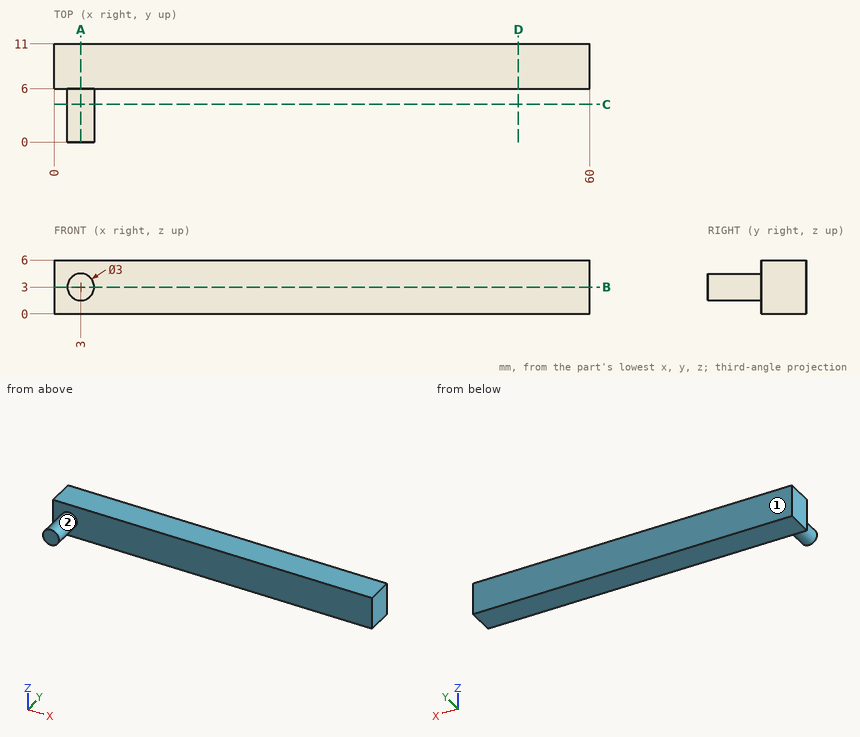
Input: dimensioned drawing with shaded views. Units: mm. Origin: part minimum x, y, z. A direction names the side the tool comes from. Give positions to 0.01 mm unless a question says otherwise; leave off trailing zeros. Order: outer loops, then holes, each group sorted by start corner. A loop starts at its lowest first (then second) coordinate and runs counter-clockwise, first axis right, second up. Notation, with made-up numbers: (-39, -15) -> (9, -15) arc R6 cw to (9, -9) -> close; hole circle Ø9 at (46, 19). An arc over 180 degrees is marked (long way). Use one line per item in the form item = value.
1) Section B-B, the plane z = 3. Return loops of the section in (x, y).
Response values:
outline = (0, 6) -> (1.5, 6) -> (1.5, 0) -> (4.5, 0) -> (4.5, 6) -> (60, 6) -> (60, 11) -> (0, 11) -> close
2) Line query: probe 1 along Y at (x, z) = (27, 1.6); probe 2 along Z at (x, y) = (4, 1.5); probe 3 along X at (y, z) = (2, 3.3). Output: solid intervals per line, ascending.
Response values:
probe_1 = 6 to 11
probe_2 = 1.88 to 4.12
probe_3 = 1.53 to 4.47
3) Section C-C, the plane y = 4.25. Return loops of the section in (x, z), and give its area (3 significant figures).
Response values:
outline = circle Ø3 at (3, 3)
area = 7.07 mm^2
4) Section D-D, the plane x = 52. Return loops of the section in (y, z), and give its area (3 significant figures).
Response values:
outline = (6, 0) -> (11, 0) -> (11, 6) -> (6, 6) -> close
area = 30.0 mm^2
5) First-contact query: pin 1 Ø3 at (x, z) = (32.5, 1.5) entering from -Y; pin 2 Ø1.5 at (y, z) = (4.5, 3) entering from -X. Flat tips, straight axial feed; report the tip coordinate or a pass-through.
Response values:
pin_1 = 6
pin_2 = 1.5
6) Section A-A, the plane x = 3. Return loops of the section in (y, z), and give its area (3 significant figures).
Response values:
outline = (0, 1.5) -> (6, 1.5) -> (6, 0) -> (11, 0) -> (11, 6) -> (6, 6) -> (6, 4.5) -> (0, 4.5) -> close
area = 48.0 mm^2
7) Reachability of the marked faces 1 and 2 from +Z, -Z, +X, -X, +Y, -Y: full face, straight path, thin tool, end or side. Return the list, or none.
Response values:
face_1 = +Z, -Z, +X, -X, +Y
face_2 = -Y
